```python
from build123d import *

# Parameters (mm, degrees)
F0_R     = 11
F1_DEPTH = 10
F2_W     = 26.7762894586
F2_H     = 3
F3_DEPTH = 11.5
F4_R     = 2
F5_DEPTH = 25
F6_R     = 4


# Not quite as in the source:
# - a feature names something its author has since deleted; it is built from what else it names


with BuildPart() as f1:
    # F0 (on Top) → F1 (new body)
    with BuildSketch(Plane.XY):
        with BuildLine():
            Line((20.8116516682, 3.3799528892), (12.8116516682, 3.3799528892))
            ThreePointArc((12.8116516682, 3.3799528892), (-13.25, 0), (12.8116516682, -3.3799528892))
            Line((12.8116516682, -3.3799528892), (12.8116516682, -3.6200471108))
            Line((12.8116516682, -3.6200471108), (20.8116516682, -3.6200471108))
            Line((20.8116516682, -3.6200471108), (20.8116516682, 3.3799528892))
        make_face()
        Circle(F0_R, mode=Mode.SUBTRACT)
    extrude(amount=F1_DEPTH)

    # F2 (on Top) → F3 (cut, symmetric)
    with BuildSketch(Plane.XY):
        with Locations((19.2577867381, 0)):
            Rectangle(F2_W, F2_H)
    extrude(amount=F3_DEPTH, both=True, mode=Mode.SUBTRACT)

    # F4 (on face) → F5 (cut)
    with BuildSketch(Plane.XZ.offset(3.6200471108)):
        with Locations((16.8116516682, 5)):
            Circle(F4_R)
    extrude(amount=-F5_DEPTH, mode=Mode.SUBTRACT)

    # F6
    f6_edges = [f1.edges().sort_by_distance(p)[0] for p in [
        (20.811652, -2.560024, 10),
        (20.811652, 2.439976, 10),
        (20.811652, 2.439976, 0),
        (20.811652, -2.560024, 0),
    ]]
    fillet(f6_edges, radius=F6_R)


solid = f1.part
```
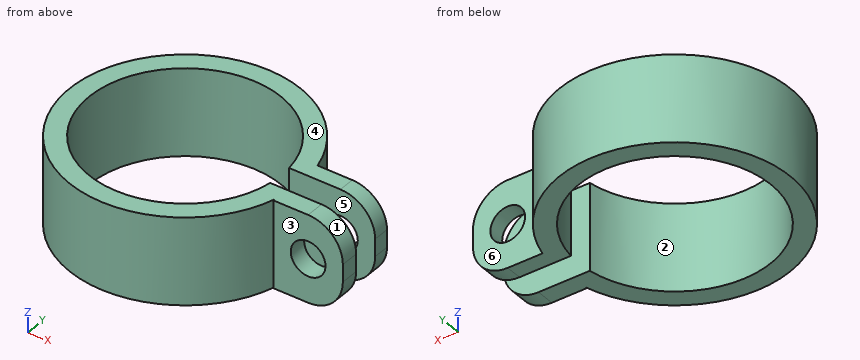
Source: CAD feature listing. Evaluate the final solid. Frame: model axes, mm. Face numbers are marked on the shaded views. A direction names the side the tool comes from. Give positions to 0.01 mm unless a question says otherwise; leave off trailing zeros. Order: outer loops, then holes, each group sorted by start corner. A loop starts at its lowest first (then second) coordinate and runs counter-clockwise, first axis right, second up. Notation, with made-up numbers: (82, 83) -> (105, 83) arc R6 ccw to (105, 94) -> close; hole circle Ø9 at (80.5, -17). An arc over 180 degrees is marked (long way). Use a Markdown table: item, result.
Q1. First-contact query: P1, Ø4, axis at x = 18, z = 4.5, coming from the -Y side; P2, Ø6, axis at x = -5.5, z = 8, coming from the +Y side; P3, Ø2.5, axis at x = 15, z = 6.5, coming from the +Y side; P4, Ø3, axis at x = -8.5, y = 5, coming from the +Z side. Flat tips, straight axial feed; report the tip coordinate or a pass-through.
A:
| item | result |
|---|---|
| P1 | y = -3.62 |
| P2 | y = 13.01 |
| P3 | y = 3.38 |
| P4 | z = 10 |
Q2. Section D-D (y = 0). Return the cut outline in (x, z).
A:
| item | result |
|---|---|
| outline | (-13.25, 0) -> (-11, 0) -> (-11, 10) -> (-13.25, 10) -> close |
Q3. Access query for the marked faces 4, 5 and 6. Directions: +Z, -Z, +X, -X, +Y, -Y. A direction counts if a zero-diameter tool reaches every point of the face in a straight line with its end or side. Return the directions, or none.
A:
| item | result |
|---|---|
| face 4 | +Z, +X, -X, +Y, -Y |
| face 5 | +Z, -Z, +X |
| face 6 | +Z, -Z, +X, +Y |
Q4. Section B-B (z = 5). Return the cut outline in (x, y).
A:
| item | result |
|---|---|
| outline | (10.9, -1.5) arc R11 cw (long way) to (10.9, 1.5) -> (14.81, 1.5) -> (14.81, 3.38) -> (12.81, 3.38) arc R13.25 ccw (long way) to (12.81, -3.38) -> (12.81, -3.62) -> (14.81, -3.62) -> (14.81, -1.5) -> close; (18.81, -3.62) -> (20.81, -3.62) -> (20.81, -1.5) -> (18.81, -1.5) -> close; (18.81, 1.5) -> (20.81, 1.5) -> (20.81, 3.38) -> (18.81, 3.38) -> close |
Q5. Material intervals for line 1 (X direction, y = -3, z = 6.75); line 2 (Y direction, x = 0, z = 7.75); line 3 (Y direction, x = -2, z = 7.75), sorted ascending. Write a range as [from, to].
A:
| item | result |
|---|---|
| line 1 | [-12.91, -10.58], [10.58, 15.84], [17.78, 20.74] |
| line 2 | [-13.25, -11], [11, 13.25] |
| line 3 | [-13.1, -10.82], [10.82, 13.1] |
Q6. Pull-direction query (Y, two-part tool) for the marked faces 1, 2 and 3; classes: +Y half, -Y half, draft (parallel to the pull), parting line (faces both ways), or undercut.
A:
| item | result |
|---|---|
| face 1 | draft |
| face 2 | undercut |
| face 3 | -Y half |
Q7. Section C-C (y = -7.5). Return the cut outline in (x, z).
A:
| item | result |
|---|---|
| outline | (-10.92, 0) -> (-8.05, 0) -> (-8.05, 10) -> (-10.92, 10) -> close; (8.05, 0) -> (10.92, 0) -> (10.92, 10) -> (8.05, 10) -> close |
Q8. Section A-A (x = 0). Return the cut outline in (y, z).
A:
| item | result |
|---|---|
| outline | (-13.25, 0) -> (-11, 0) -> (-11, 10) -> (-13.25, 10) -> close; (11, 0) -> (13.25, 0) -> (13.25, 10) -> (11, 10) -> close |
